Part print with two shaded views. Sizes in mm from the minimum x, y, z corner. A direction names the side the tool comes from. Coordinates: 2 decimals unless noted, no trailing zeros. Loops run counter-clockwise (first coordinate to the right, second up) from the corner with the lowest first, then second, coordinate; pieces in that order, holes last.
Item 1: Cut at D-D (x = 26). List the corners of the cut face in (y, z).
Item 2: Cut at C-C (y = 6.5). List the corners of the cut face in (x, z), and give its area (3 significant figures).
Item 3: Cut at A-A (y = 13). List the corners of the cut face in (x, z), and give its area (3 significant figures).
Item 4: Cut at B-B (z = 4.25). List the corners of the cut face in (x, y).
Item 5: Mould opens along X. For the marked faces 1, 2 and 3 say: released by +X, released by -X, zero draft, split by the parting line, or undercut.
Item 6: Drill centre lines: line 1 along X through (y, z) = (9, 11.75); line 2 along Y through (x, z) = (32, 20.5); line 3 along Y through (x, z) = (36.5, 3.25). Where is each one in solid material? Low to high.
Item 7: 3-axis set-ups, long thin cutter, end or side, ignore diameter. For the marked faces 4 and 5: which of +Z, -Z, +X, -X, +Y, -Y reach the whole face in a straight line?
Item 8: Flat gauge pins, fed straight in: pin 1 (8 mm diameter, centred on x = 17, z = 19.5, fed in from -Y); pin 2 (8 mm diameter, centred on y = 14, z = 19, fed in from +X); pin 3 (2 mm diameter, centred on y = 1.5, z = 7, fed in from -X). Where does each tip first touch, or does it go through?
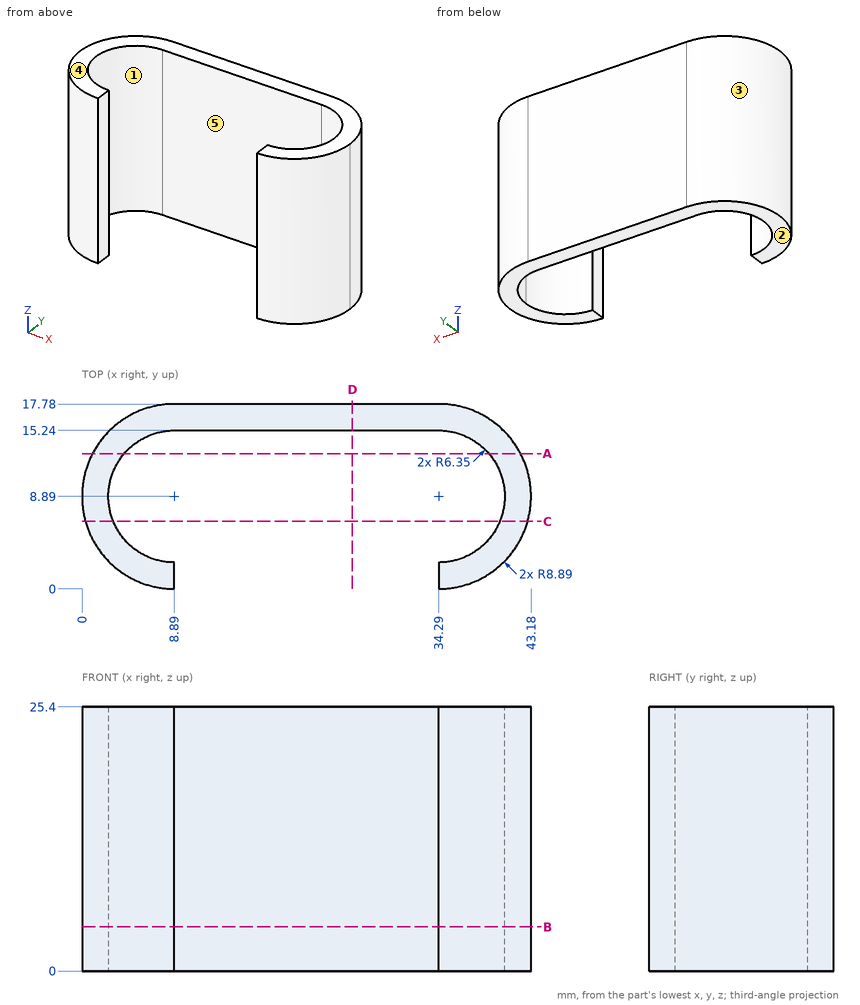
Filled sheet:
1. outline: (15.24, 0) - (17.78, 0) - (17.78, 25.4) - (15.24, 25.4) - close
2. outline: (0.33, 0) - (3.01, 0) - (3.01, 25.4) - (0.33, 25.4) - close; (40.17, 0) - (42.85, 0) - (42.85, 25.4) - (40.17, 25.4) - close
2. area: 136 mm2
3. outline: (1.01, 0) - (4.05, 0) - (4.05, 25.4) - (1.01, 25.4) - close; (39.13, 0) - (42.17, 0) - (42.17, 25.4) - (39.13, 25.4) - close
3. area: 155 mm2
4. outline: (8.89, 0) - (8.89, 2.54) arc R6.35 cw to (8.89, 15.24) - (34.29, 15.24) arc R6.35 cw to (34.29, 2.54) - (34.29, 0) arc R8.89 ccw to (43.18, 8.89) arc R8.89 ccw to (34.29, 17.78) - (8.89, 17.78) arc R8.89 ccw to start
5. face 1: undercut
5. face 2: zero draft
5. face 3: released by -X
6. line 1: x = 0 to 2.54, 40.64 to 43.18
6. line 2: y = 15.24 to 17.78
6. line 3: y = 0.28 to 2.94, 14.84 to 17.5
7. face 4: +Z, +X, -X, +Y, -Y
7. face 5: +Z, -Z, -Y
8. pin 1: stops at y = 15.24
8. pin 2: stops at x = 43.11
8. pin 3: stops at x = 2.71
